The model under review builds one solid part; all positions refer to its coordinate system, in mm. A direction names the side the tool comes from. Give positions to 0.01 mm unless a question says otherwise; leave off trailing zeros. Order: outer loops, then holes, each group sorted by start corner. A loop starts at its lowest first (then second) coordinate and runs counter-clockwise, first axis right, second up. Notation, with made-up numbers: (13.25, 68) - (71.25, 68) arc R19 cw to (71.25, 97) - close; hole circle Ø10 at (11.5, -10). An arc over 180 degrees is marked (long way). Put each result on its own line as item: value.
```python
from build123d import *

# Parameters (mm, degrees)
SKETCH_R         = 1.75
PAD004_DEPTH     = 1.5
SKETCH001001_R   = 1.75
SKETCH001001_W   = 98.5
SKETCH001001_H   = 39
PAD005_DEPTH     = 1.5
SKETCH003002_R   = 1.75
PAD001_DEPTH     = 1.5
SKETCH003004_R   = 1.75
PAD002_DEPTH     = 1.5
SKETCH003003_W   = 3
SKETCH003003_H   = 9.6
SKETCH003003_W_2 = 14.6
SKETCH003003_H_2 = 3
PAD_DEPTH        = 1.5
FILLET_R         = 5


with BuildPart() as pad004:
    # Sketch → Pad004 (new body, symmetric)
    with BuildSketch(Plane.XY):
        with Locations((-108.5, 38.5)):
            Circle(SKETCH_R)
        with Locations((-108.5, -38.5)):
            Circle(SKETCH_R)
        with Locations((108.5, 38.5)):
            Circle(SKETCH_R)
        with Locations((108.5, -38.5)):
            Circle(SKETCH_R)
    extrude(amount=PAD004_DEPTH, both=True)


with BuildPart() as pad005:
    # Sketch001001 → Pad005 (new body, symmetric)
    with BuildSketch(Plane.XY):
        with Locations((46.5, 27.5)):
            Circle(SKETCH001001_R)
        with Locations((-46.5, 27.5)):
            Circle(SKETCH001001_R)
        with Locations((-46.5, -27.5)):
            Circle(SKETCH001001_R)
        with Locations((46.5, -27.5)):
            Circle(SKETCH001001_R)
        Rectangle(SKETCH001001_W, SKETCH001001_H)
    extrude(amount=PAD005_DEPTH, both=True)


with BuildPart() as pad001:
    # Sketch003002 → Pad001 (new body, symmetric)
    with BuildSketch(Plane.XY):
        with Locations((-70, -25)):
            Circle(SKETCH003002_R)
        with Locations((-70, -5)):
            Circle(SKETCH003002_R)
        with Locations((-60, -5)):
            Circle(SKETCH003002_R)
        with Locations((-60, -25)):
            Circle(SKETCH003002_R)
    extrude(amount=PAD001_DEPTH, both=True)


with BuildPart() as pad002:
    # Sketch003004 → Pad002 (new body, symmetric)
    with BuildSketch(Plane.XY):
        with Locations((-70, 5)):
            Circle(SKETCH003004_R)
        with Locations((-70, 25)):
            Circle(SKETCH003004_R)
        with Locations((-60, 25)):
            Circle(SKETCH003004_R)
        with Locations((-60, 5)):
            Circle(SKETCH003004_R)
    extrude(amount=PAD002_DEPTH, both=True)


with BuildPart() as fillet_body:
    # Sketch003003 → Pad (new body, symmetric)
    with BuildSketch(Plane.XY):
        Polygon((-120, 50), (120, 50), (120, -50), (50, -50), (50, -32), (-50, -32), (-50, -50), (-120, -50), align=None)
        with Locations((108.5, -25)):
            Rectangle(SKETCH003003_W, SKETCH003003_H, mode=Mode.SUBTRACT)
        with Locations((108.5, 25)):
            Rectangle(SKETCH003003_W, SKETCH003003_H, mode=Mode.SUBTRACT)
        with Locations((-108.5, 25)):
            Rectangle(SKETCH003003_W, SKETCH003003_H, mode=Mode.SUBTRACT)
        with Locations((-108.5, -25)):
            Rectangle(SKETCH003003_W, SKETCH003003_H, mode=Mode.SUBTRACT)
        with Locations((-77.5, 38.5)):
            Rectangle(SKETCH003003_W_2, SKETCH003003_H_2, mode=Mode.SUBTRACT)
        with Locations((-32.5, 38.5)):
            Rectangle(SKETCH003003_W_2, SKETCH003003_H_2, mode=Mode.SUBTRACT)
        with Locations((32.5, 38.5)):
            Rectangle(SKETCH003003_W_2, SKETCH003003_H_2, mode=Mode.SUBTRACT)
        with Locations((77.5, 38.5)):
            Rectangle(SKETCH003003_W_2, SKETCH003003_H_2, mode=Mode.SUBTRACT)
    extrude(amount=PAD_DEPTH, both=True)

    # Cut: cut Pad002
    add(pad002.part, mode=Mode.SUBTRACT)

    # Cut001: cut Pad001
    add(pad001.part, mode=Mode.SUBTRACT)

    # Cut002: cut Pad005
    add(pad005.part, mode=Mode.SUBTRACT)

    # Cut003: cut Pad004
    add(pad004.part, mode=Mode.SUBTRACT)

    # Fillet
    fillet_edges = [fillet_body.edges().sort_by_distance(p)[0] for p in [
        (50, -50, 0),
        (120, -50, 0),
        (50, -32, 0),
        (120, 50, 0),
        (-50, -32, 0),
        (-120, 50, 0),
        (-50, -50, 0),
        (-120, -50, 0),
    ]]
    fillet(fillet_edges, radius=FILLET_R)


solid = fillet_body.part
```
(1) Take a section at C-C, the plane z = 0.55. Count the separate pieces of the cut face and the enclosed holes in it, then the cut area to 3 significant figures.
The answers:
separate pieces: 1
enclosed holes: 25
area: 17,900 mm^2
(2) Wall thickness on L1, parallel to Y at x = -60, z = -0.8; L2, parallel to X at y = 29.5, z = 0.75; L3, parallel to Y at x = 8.5, z = 0.6: over which ranges is each line inside the solid? List them lowest first.
The answers:
L1: -50 to -26.75, -23.25 to -6.75, -3.25 to 3.25, 6.75 to 23.25, 26.75 to 50
L2: -120 to -110, -107 to 107, 110 to 120
L3: -32 to -19.5, 19.5 to 50
(3) Take a section at B-B, the plane y = -13.5. Write out the cut boundary in (x, z), then the cut area to 4 significant figures.
The answers:
outline: (-120, -1.5) - (-49.25, -1.5) - (-49.25, 1.5) - (-120, 1.5) - close; (49.25, -1.5) - (120, -1.5) - (120, 1.5) - (49.25, 1.5) - close
area: 424.5 mm^2
(4) Take a section at A-A, the plane x = 23. Write out the cut boundary in (y, z), then the cut area to 3 significant figures.
The answers:
outline: (-32, -1.5) - (-19.5, -1.5) - (-19.5, 1.5) - (-32, 1.5) - close; (19.5, -1.5) - (50, -1.5) - (50, 1.5) - (19.5, 1.5) - close
area: 129 mm^2
(5) The part is to be moulded in two halves that separate along X. For faces 1 (the cylindrical face through (119, -48, 0)), 2 (the cylindrical face through (-49, -34, 0)), 3 (the flat face through (2, 23, -1.5)), say which applies: pulls with the +X half, pulls with the -X half, needs draft (parallel to the pull), parting line crosses it, or undercut.
The answers:
face 1: pulls with the +X half
face 2: undercut
face 3: needs draft
(6) For faces 4 (the cylindrical face through (52, -49, 0)), 5 (the cylindrical face through (118, 49, 0)), list the 3-axis set-ups (+Z, -Z, +X, -X, +Y, -Y) from which the entire face can be reached by the end or side of a thin tool; tool diameter is ignored.
The answers:
face 4: +Z, -Z, -Y
face 5: +Z, -Z, +X, +Y
(7) Clearance check with flat-ended pins moving along their axes: pin 1 Ø2 at (x, y) = (-70, 25) entering from +Z; pin 2 Ø1.5 at (x, z) = (46, -1) entering from -Y. State where each tip first meets the part, or that it passes through.
The answers:
pin 1: through
pin 2: y = -32.32
